```python
from build123d import *

# Parameters (mm, degrees)
EXTRUDE_1_DEPTH      = 10
EXTRUDE_1_DEPTH_BACK = 10
SKETCH_3_R           = 4
EXTRUDE_2_DEPTH      = 8
SKETCH_2_R           = 2
CUT_EXTRUDE_1_DEPTH  = 10
SKETCH_4_R           = 4.2
SKETCH_4_R_2         = 2
CUT_EXTRUDE_2_DEPTH  = 2.7


with BuildPart() as part:
    # Эскиз1 → Бобышка-Вытянуть1 (new body, two sides)
    with BuildSketch(Plane(origin=(-110, 0, 0), x_dir=(0, 0, -1), z_dir=(1, 0, 0))) as extrude_1_sk:
        Polygon((-4.2, -5), (-4.2, -1.3625), (4.2, -1.3625), (4.2, -5), (10, -5), (10, 3), (-10, 3), (-10, -5), align=None)
    extrude(amount=EXTRUDE_1_DEPTH)
    extrude(extrude_1_sk.sketch, amount=-EXTRUDE_1_DEPTH_BACK)

    # Эскиз3 → Бобышка-Вытянуть2 (add, through all)
    with BuildSketch(Plane(origin=(0, 3, 0), x_dir=(1, 0, 0), z_dir=(0, 1, 0))):
        with Locations((-110, -9)):
            Circle(SKETCH_3_R)
        with Locations((-110, 9)):
            Circle(SKETCH_3_R)
    extrude(amount=-EXTRUDE_2_DEPTH)

    # Эскиз2 → Вырез-Вытянуть1 (cut)
    with BuildSketch(Plane(origin=(0, 3, 0), x_dir=(1, 0, 0), z_dir=(0, 1, 0))):
        with Locations((-110, -9)):
            Circle(SKETCH_2_R)
        with Locations((-110, 9)):
            Circle(SKETCH_2_R)
    extrude(amount=-CUT_EXTRUDE_1_DEPTH, mode=Mode.SUBTRACT)

    # Эскиз4 → Вырез-Вытянуть2 (cut)
    with BuildSketch(Plane.XZ.offset(5)):
        with Locations((-110, 9)):
            Circle(SKETCH_4_R)
        with Locations((-110, 9)):
            Circle(SKETCH_4_R_2, mode=Mode.SUBTRACT)
        with Locations((-110, -9)):
            Circle(SKETCH_4_R)
        with Locations((-110, -9)):
            Circle(SKETCH_4_R_2, mode=Mode.SUBTRACT)
    extrude(amount=-CUT_EXTRUDE_2_DEPTH, mode=Mode.SUBTRACT)


solid = part.part
```
Work out the finished part from the listing and answer in its coordinate system (mm). A direction names the side the tool comes from. Give positions to 0.01 mm unless a question says otherwise; leave off trailing zeros. Order: outer loops, then holes, each group sorted by start corner. A loop starts at its lowest first (then second) coordinate and runs counter-clockwise, first axis right, second up. Notation, with made-up numbers: (86, 53) - (92, 53) arc R26 cw to (92, 82) - close; hole circle Ø4 at (57.5, 20). An arc over 180 degrees is marked (long way). One line per item, written item: value. Start each with the question number.
1. Each of these flat-tipped pins is pushed along its axis until it touches: pin 1 Ø1.8 at (x, y) = (-106, -3.5) entering from +Z; pin 2 Ø7.5 at (x, z) = (-110, 9) entering from -Y; pin 3 Ø4 at (x, y) = (-107, -2.5) entering from -Z. Where does it stop, or does it pass through?
2. Section C-C, the plane y = 1.75 is taken. Write down the section's boundary in (x, z), then the cut area to 3 significant figures.
3. Section A-A, the plane z = 9 is taken. Write down the section's boundary in (x, y), then the cut area to 3 significant figures.
4. Which of the six approach directions +Z, -Z, +X, -X, +Y, -Y give full straight-line access (tool end or side, diameter ignored) to faces 5 (the face through (-110, -3, -4.2)), 6 (the face through (-103, -1, 10)), 7 (the face through (-117, -1, -10)), 8 (the face through (-110.1, -3.7, 4.8))?
5. Consider line 1 (Z direction, x = -110, y = -0.3); line 2 (Z direction, x = -110, y = -4); line 3 (X direction, y = 0.9, z = -9). Determine where each line is inside the solid, lowest interval first.
6. For a pull along Z with two mould halves and no side action, classify faces 1 (the face through (-103, -1, -10)), 2 (the face through (-112, 0, 9)), 3 (the face through (-109.9, -3.7, -4.8)), 4 (the face through (-109.9, -5, -4.5)) as released by +Z, released by -Z, zero draft, split by the parting line, or undercut.
7. Section B-B, the plane x = -104.75 is taken. Write down the section's boundary in (y, z), then the cut area to 3 significant figures.
8. Section D-D, the plane x = -110 is taken. Write down the section's boundary in (y, z).
Filled sheet:
1. pin 1: z = 10
1. pin 2: y = -2.3
1. pin 3: z = -12.87
2. outline: (-120, -10) - (-113.87, -10) arc R4 ccw to (-106.13, -10) - (-100, -10) - (-100, 10) - (-106.13, 10) arc R4 ccw to (-113.87, 10) - (-120, 10) - close; hole circle Ø4 at (-110, -9); hole circle Ø4 at (-110, 9)
2. area: 409 mm²
3. outline: (-120, -5) - (-114.2, -5) - (-114.2, -2.3) - (-112, -2.3) - (-112, 3) - (-120, 3) - close; (-108, -2.3) - (-105.8, -2.3) - (-105.8, -5) - (-100, -5) - (-100, 3) - (-108, 3) - close
3. area: 116 mm²
4. face 5: +X, -X, -Y
4. face 6: +Z, +X, +Y, -Y
4. face 7: -Z, -X, +Y, -Y
4. face 8: -Y
5. line 1: -13 to -11, -7 to 7, 11 to 13
5. line 2: -4.8 to -4.2, 4.2 to 4.8
5. line 3: -120 to -112, -108 to -100
6. face 1: released by -Z
6. face 2: undercut
6. face 3: undercut
6. face 4: zero draft
7. outline: (-5, -10) - (3, -10) - (3, 10) - (-5, 10) - (-5, 4.2) - (-1.36, 4.2) - (-1.36, -4.2) - (-5, -4.2) - close
7. area: 129 mm²
8. outline: (-5, -4.8) - (-2.3, -4.8) - (-2.3, -7) - (3, -7) - (3, 7) - (-2.3, 7) - (-2.3, 4.8) - (-5, 4.8) - (-5, 4.2) - (-1.36, 4.2) - (-1.36, -4.2) - (-5, -4.2) - close; (-2.3, -13) - (3, -13) - (3, -11) - (-2.3, -11) - close; (-2.3, 11) - (3, 11) - (3, 13) - (-2.3, 13) - close
